```python
from build123d import *

# Parameters (mm, degrees)
SKETCH1_R           = 22.225
SKETCH1_R_2         = 5.1308
BOSS_EXTRUDE1_DEPTH = 31.75


with BuildPart() as part:
    # Sketch1 → Boss-Extrude1 (new body)
    with BuildSketch(Plane(origin=(0, 0, 0), x_dir=(1, 0, 0), z_dir=(0, 1, 0))):
        Polygon((-30.48, 80.01), (50.8, 80.01), (50.8, -53.34), (-50.8, -53.34), (-50.8, 44.81472759), align=None)
        with Locations(Location((0, 0, 0), (0, 0, 270))):
            Circle(SKETCH1_R, mode=Mode.SUBTRACT)
        with Locations(Location((35.56, 38.1, 0), (0, 0, 270))):
            Circle(SKETCH1_R_2, mode=Mode.SUBTRACT)
        with Locations(Location((-35.56, 38.1, 0), (0, 0, 270))):
            Circle(SKETCH1_R_2, mode=Mode.SUBTRACT)
        with Locations(Location((-35.56, -38.1, 0), (0, 0, 270))):
            Circle(SKETCH1_R_2, mode=Mode.SUBTRACT)
        with Locations(Location((35.56, -38.1, 0), (0, 0, 270))):
            Circle(SKETCH1_R_2, mode=Mode.SUBTRACT)
        with BuildLine():
            Line((-15.24, 65.0875), (15.24, 65.0875))
            ThreePointArc((15.24, 65.0875), (23.1775, 57.15), (15.24, 49.2125))
            Line((15.24, 49.2125), (-15.24, 49.2125))
            ThreePointArc((-15.24, 49.2125), (-23.1775, 57.15), (-15.24, 65.0875))
        make_face(mode=Mode.SUBTRACT)
    extrude(amount=BOSS_EXTRUDE1_DEPTH)


solid = part.part
```
The listing builds one solid part. Answer for the finished solid, in the listing's coordinates (mm). A direction names the side the tool comes from. Coordinates: 2 decimals unless noted, no trailing zeros. Write each loop counter-clockwise with the first axis right and the second up, starting at its lowest first coordinate (ties: lowest second). Pieces come first, ordered by that corner, then holes. Notation, with made-up numbers: (73.5, 7) - (110.5, 7) arc R16 cw to (110.5, 12) - close; hole circle Ø2 at (55, 27.5). An arc over 180 degrees is marked (long way). Return JSON: item names as keys, results as strings. Group by question number.
1. A cutting plane is placed at C-C, the plane z = 0. Determine the outline of the cut face in (x, y) (3 decimals), plus the area to 3 significant figures.
2. Determine the mould class of faces 3 (the flat face through (10, 16, -80.01)), 4 (the flat face through (1, 31.75, -29)), 5 (the flat face through (0, 16, -65.088)), 6 (the cylindrical face through (-30.473, 15.653, -38.768)) for opening direction Z: released by +Z, released by -Z, zero draft, split by the parting line, or undercut.
3. Which of the six approach directions +Z, -Z, +X, -X, +Y, -Y give full straight-line access (tool end or side, diameter ignored) to faces 1 (the flat face through (1, 0, -29)), 2 (the flat face through (0, 16, -49.212))?
4. A cutting plane is placed at A-A, the plane z = -38.1. Determine the outline of the cut face in (x, y).
5. A cutting plane is placed at B-B, the plane x = 0. Give the number of separate pieces and of enclosed holes in the cut face, plus the area to 3 significant figures.
6. Straight lines are drawn through the part: L1, parallel to X at y = 23, z = -38.1; L2, parallel to Z at x = -32, y = 15.5; L3, parallel to Z at x = 34.5, y = 23. For each, find the intervals that lie inside material, in ascending order.
Ans:
{
 "1": {"outline": "(-50.8, 0) - (-22.225, 0) - (-22.225, 31.75) - (-50.8, 31.75) - close; (22.225, 0) - (50.8, 0) - (50.8, 31.75) - (22.225, 31.75) - close", "area": "1,810 mm²"},
 "2": {"face 3": "released by -Z", "face 4": "zero draft", "face 5": "undercut", "face 6": "undercut"},
 "3": {"face 1": "+Z, -Z, +X, -X, -Y", "face 2": "+Y, -Y"},
 "4": {"outline": "(-50.8, 0) - (-40.69, 0) - (-40.69, 31.75) - (-50.8, 31.75) - close; (-30.43, 0) - (30.43, 0) - (30.43, 31.75) - (-30.43, 31.75) - close; (40.69, 0) - (50.8, 0) - (50.8, 31.75) - (40.69, 31.75) - close"},
 "5": {"separate pieces": "3", "enclosed holes": "0", "area": "2,320 mm²"},
 "6": {"L1": "-50.8 to -40.69, -30.43 to 30.43, 40.69 to 50.8", "L2": "-77.38 to -41.79, -34.41 to 34.41, 41.79 to 53.34", "L3": "-80.01 to -43.12, -33.08 to 33.08, 43.12 to 53.34"}
}
